Read the model definition and answer for the solid it produces. Units are mm, in the model's axes. A direction names the side the tool comes from. Give positions to 0.01 mm unless a question says otherwise; leave off trailing zeros. Write each loop counter-clockwise with the first axis right and the second up, starting at its lowest first coordinate (ties: lowest second). Pieces come first, ordered by that corner, then holes. Notation, with made-up numbers: (78.25, 10) -> (92.25, 10) arc R18 cw to (92.25, 34) -> close; hole circle Ø3 at (-31, 20). An arc over 180 degrees is marked (long way). Answer as CSV lines item,"result". Start each with the question number.
1. For a pull along Y with two mould halves and no side action, classify faces 6 (the cylindrical face through (4.42, -12.11, 5.07)), 7 (the flat face through (0, -3, 5)), 8 (the cylindrical face through (2.62, 14.77, 4.93)) as pulls with the +Y half, pulls with the -Y half, needs draft (parallel to the pull), parting line crosses it, or undercut.
2. The part is cut by section A-A, the plane y = 2. Determine the outline of the cut face in (x, z), and give its area (3 significant figures).
3. The part is cut by section C-C, the plane x = 10. Determine the outline of the cut face in (y, z).
4. The part is cut by section B-B, the plane x = 3. Determine the outline of the cut face in (y, z).
5. Given pin 1 (1.3 mm diameter, centred on y = -4, z = 3, fed in from +X); pin 2 (8 mm diameter, centred on x = 9.5, y = 10, fed in from -Z); pin 3 (2 mm diameter, centred on y = -7.5, z = 7.5, fed in from +X); pin 4 (2 mm diameter, centred on y = 2, z = 5, fed in from -X), each flat-ended and moving along its own axis, determine where each tip first touches the part or whether it passes through.
6. A tool of negligible diameter and unlimited length cuts with its end or side. For faces 1 (the flat face through (13.568, 3.564, 5.07)), 2 (the flat face through (-1.154, 13.98, 5.07)), 3 (the cylindrical face through (14.1, 5.12, 4.93)), 4 (the flat face through (-11.512, 7.968, 5.07)), 5 (the flat face through (-12.656, -5.986, 5.07)), from which of +Z, -Z, +X, -X, +Y, -Y can it reach the whole face along a straight path? Write none if from no direction.
7. The part is cut by section D-D, the plane y = 11.25. Determine the outline of the cut face in (x, z).
8. Find the intervals of material crossed by line 1 (Y direction, x = 12, z = 1.5); line 2 (X direction, y = 12.5, z = 3.25); line 3 (Y direction, x = 11, z = 3.75), in increasing order.
from build123d import *

# Parameters (mm, degrees)
F0_R     = 15
F1_DEPTH = 10
F3_DEPTH = 10.001
F4_COUNT = 18


with BuildPart() as f1:
    # F0 (on Top) → F1 (new body)
    with BuildSketch(Plane.XY):
        Circle(F0_R)
        with BuildLine():
            ThreePointArc((1.5, 4.7696960071), (5, 0), (1.5, -4.7696960071))
            Line((1.5, -4.7696960071), (1.5, -3.2))
            ThreePointArc((1.5, -3.2), (1.4414213562, -3.0585786438), (1.3, -3))
            Line((1.3, -3), (-1.3, -3))
            ThreePointArc((-1.3, -3), (-1.4414213562, -3.0585786438), (-1.5, -3.2))
            Line((-1.5, -3.2), (-1.5, -4.7696960071))
            ThreePointArc((-1.5, -4.7696960071), (-5, 0), (-1.5, 4.7696960071))
            Line((-1.5, 4.7696960071), (-1.5, 3.2))
            ThreePointArc((-1.5, 3.2), (-1.4414213562, 3.0585786438), (-1.3, 3))
            Line((-1.3, 3), (1.3, 3))
            ThreePointArc((1.3, 3), (1.4414213562, 3.0585786438), (1.5, 3.2))
            Line((1.5, 3.2), (1.5, 4.7696960071))
        make_face(mode=Mode.SUBTRACT)
    extrude(amount=F1_DEPTH)

    # F2 (on face) → F3 (cut, through all)
    with BuildSketch(Plane.XY.offset(10)):
        with BuildLine():
            ThreePointArc((0.6031215444, 12.8775082637), (0.7234998321, 12.9107243291), (0.8007100133, 13.0088712958))
            Line((0.8007100133, 13.0088712958), (1.4981238267, 14.925))
            ThreePointArc((1.4981238267, 14.925), (0, 15), (-1.4981238267, 14.925))
            Line((-1.4981238267, 14.925), (-0.8007100133, 13.0088712958))
            ThreePointArc((-0.8007100133, 13.0088712958), (-0.7234998321, 12.9107243291), (-0.6031215444, 12.8775082637))
            ThreePointArc((-0.6031215444, 12.8775082637), (0, 12.8920669658), (0.6031215444, 12.8775082637))
        make_face()
    f3 = extrude(amount=-F3_DEPTH, mode=Mode.SUBTRACT)

    # F4: F3 ×18 about axis
    f4_axis = Axis((0, 0, 0), (0, 0, -1))
    for i in range(1, F4_COUNT):
        add(f3.rotate(f4_axis, i * 360 / F4_COUNT), mode=Mode.SUBTRACT)


solid = f1.part
Results found:
1,face 6,"pulls with the -Y half"
1,face 7,"undercut"
1,face 8,"pulls with the +Y half"
2,outline,"(-12.74, 0) -> (-4.58, 0) -> (-4.58, 10) -> (-12.74, 10) -> close; (4.58, 0) -> (12.74, 0) -> (12.74, 10) -> (4.58, 10) -> close"
2,area,"163 mm²"
3,outline,"(-10.04, 0) -> (10.04, 0) -> (10.04, 10) -> (-10.04, 10) -> close"
4,outline,"(-14.7, 0) -> (-4, 0) -> (-4, 10) -> (-14.7, 10) -> close; (4, 0) -> (14.7, 0) -> (14.7, 10) -> (4, 10) -> close"
5,pin 1,"stops at x = 14.44"
5,pin 2,"stops at z = 0"
5,pin 3,"stops at x = 11.96"
5,pin 4,"stops at x = -14.97"
6,face 1,"+Z, -Z, +X"
6,face 2,"+Z, -Z, +Y"
6,face 3,"+Z, -Z, +X, +Y"
6,face 4,"+Z, -Z, -X"
6,face 5,"+Z, -Z"
7,outline,"(-8.03, 0) -> (8.03, 0) -> (8.03, 10) -> (-8.03, 10) -> close"
8,line 1,"y = -9 to -8.55, -5.87 to 5.87, 8.55 to 9"
8,line 2,"x = -8.29 to -5.66, -3.7 to 3.7, 5.66 to 8.29"
8,line 3,"y = -10.2 to -7.36, -6.72 to 6.72, 7.36 to 10.2"
